Autodesk Inventor part; units mm, degrees
ref_plane "YZ Plane" through (0, 0, 0) normal (1, 0, 0) x (0, 1, 0)
ref_plane "XZ Plane" through (0, 0, 0) normal (0, 1, 0) x (-1, 0, 0)
ref_plane "XY Plane" through (0, 0, 0) normal (0, 0, 1) x (1, 0, 0)
sketch "Sketch1" plane through (0, 0, 0) normal (0, 1, 0) x (-1, 0, 0)
  line L0 (0, 0) -> (13, 0)
  line L1 (13, 0) -> (13, -13)
  line L2 (13, -13) -> (0, -13)
  line L3 (0, -13) -> (0, 0)
  line L4 (13, -13) -> (58.2, -13)
  line L5 (58.2, -13) -> (58.2, -73.6)
  line L6 (58.2, -73.6) -> (13, -73.6)
  line L7 (13, -73.6) -> (13, -13)
  line L8 (58.2, -73.6) -> (71.2, -73.6)
  line L9 (71.2, -73.6) -> (71.2, -86.6)
  line L10 (71.2, -86.6) -> (58.2, -86.6)
  line L11 (58.2, -86.6) -> (58.2, -73.6)
  line L12 (0, 0) -> (71.2, 0)
  line L13 (71.2, 0) -> (71.2, -86.6)
  line L14 (71.2, -86.6) -> (0, -86.6)
  line L15 (0, -86.6) -> (0, 0)
  line L16 (58.2, -13) -> (61.2, -13)
  line L17 (61.2, -13) -> (61.2, -10)
  line L18 (61.2, -10) -> (58.2, -10)
  line L19 (58.2, -10) -> (58.2, -13)
  line L20 (13, -73.6) -> (10, -73.6)
  line L21 (10, -73.6) -> (10, -76.6)
  line L22 (10, -76.6) -> (13, -76.6)
  line L23 (13, -76.6) -> (13, -73.6)
  line L24 (61.2, -10) -> (10, -10)
  line L25 (10, -10) -> (10, -76.6)
  line L26 (10, -76.6) -> (61.2, -76.6)
  line L27 (61.2, -76.6) -> (61.2, -10)
  dimension "d0" = 13
  dimension "d1" = 13
  dimension "d2" = 45.2
  dimension "d3" = 60.6
  dimension "d4" = 13
  dimension "d5" = 13
  dimension "d6" = 3
  dimension "d7" = 3
  dimension "d8" = 3
  dimension "d9" = 3
extrude "Extrusion1" add sketch "Sketch1" along normal blind 3 contours L0 L1 L24 L25 L2 L3 | L12 L13 L8 L27 L17 L18 L24 L1 | L2 L25 L21 L22 L26 L11 L14 L15 | L9 L10 L11 L26 L27 L8
fillet "Fillet1" radius 10.58 4 edges at (0, 1.5, 0) (0, 1.5, -86.6) (-71.2, 1.5, -86.6) (-71.2, 1.5, 0)
fillet "Fillet2" radius 10.58 4 edges at (-61.2, 1.5, -76.6) (-61.2, 1.5, -10) (-10, 1.5, -10) (-10, 1.5, -76.6)
properties part number "Airpods Pro Top"
Verification items for the finished model (mm, model axes). A direction names the side the tool comes from. Give positions to 0.01 mm unless a question says otherwise; leave off trailing zeros. Order: outer loops, then holes, each group sorted by start corner. A loop starts at its lowest first (then second) coordinate and runs counter-clockwise, first axis right, second up. Notation, with made-up numbers: (-32.5, 62) -> (5.5, 62) arc R16 ccw to (5.5, 75) -> close; hole circle Ø10 at (-36, -4.75). An arc over 180 degrees is marked (long way). Use a Markdown table: item, result.
1) Material ranges on probe 1 along Z at (x, y) = (-27.5, 1.1); probe 2 along X at (y, z) = (1.4, -36); probe 3 along X at (y, z) = (2.45, -16), recorded low to high.
Results:
| item | result |
|---|---|
| probe 1 | -86.6 to -76.6, -10 to 0 |
| probe 2 | -71.2 to -61.2, -10 to 0 |
| probe 3 | -71.2 to -60.16, -11.04 to 0 |
2) Section check C-C, the plane y = 1. Record the boundary of the cut face in (x, z), then the cut area to 3 significant figures.
Results:
| item | result |
|---|---|
| outline | (-71.2, -76.02) arc R10.58 ccw to (-60.62, -86.6) -> (-10.58, -86.6) arc R10.58 ccw to (0, -76.02) -> (0, -10.58) arc R10.58 ccw to (-10.58, 0) -> (-60.62, 0) arc R10.58 ccw to (-71.2, -10.58) -> close; hole (-61.2, -66.02) arc R10.58 ccw to (-50.62, -76.6) -> (-20.58, -76.6) arc R10.58 ccw to (-10, -66.02) -> (-10, -20.58) arc R10.58 ccw to (-20.58, -10) -> (-50.62, -10) arc R10.58 ccw to (-61.2, -20.58) -> close |
| area | 2,760 mm² |
3) Mould release check, pull along X, two halves, no side actions. Record for faces 3 (the flat face through (-36, 1, -10)), 4 (the cylindrical face through (-68, 2, -3)), 5 (the flat face through (0, 1, -44)): pulls with the +X half, pulls with the -X half, needs draft (parallel to the pull), parting line crosses it, or undercut.
Results:
| item | result |
|---|---|
| face 3 | undercut |
| face 4 | pulls with the -X half |
| face 5 | pulls with the +X half |
4) Section check B-B, the plane z = -57.5. Record the boundary of the cut face in (x, y).
Results:
| item | result |
|---|---|
| outline | (-71.2, 0) -> (-61.2, 0) -> (-61.2, 3) -> (-71.2, 3) -> close; (-10, 0) -> (0, 0) -> (0, 3) -> (-10, 3) -> close |
5) Section check A-A, the plane x = -36. Record the boundary of the cut face in (y, z), then the cut area to 3 significant figures.
Results:
| item | result |
|---|---|
| outline | (0, -86.6) -> (3, -86.6) -> (3, -76.6) -> (0, -76.6) -> close; (0, -10) -> (3, -10) -> (3, 0) -> (0, 0) -> close |
| area | 60.0 mm² |
6) Tool access check on faces 1 (the flat face through (-35, 1, 0)), 2 (the flat face through (-61.2, 1, -44)). Record the directions out of +Z, -Z, +X, -X, +Y, -Y that give a thin tool (end or side, any length) a straight path to the whole face; none if there is none.
Results:
| item | result |
|---|---|
| face 1 | +Z, +X, -X, +Y, -Y |
| face 2 | +Y, -Y |
